Read the model definition and answer for the solid it produces. Units are mm, in the model's axes. Face numbers are marked on the shaded views. A direction names the side the tool comes from. Coordinates: 2 decimals unless noted, no trailing zeros. Write each loop counter-clockwise with the first axis right and the second up, starting at its lowest first coordinate (ties: lowest second). Pieces come first, ordered by that corner, then holes.
Item 1: Section A-A (y = 0) is taken. Give the vertices of the cut face in (x, z) (3 decimals).
Item 2: Section D-D (y = 10.5) is taken. Give the vertices of the cut face in (x, z).
Item 3: Section B-B (x = -9) is taken. Give the vertices of the cut face in (y, z), then the cut area to 3 significant figures.
Item 4: Each of these flat-tipped pins is pushed along its axis until it touches: P1, Ø8, axis at x = -6, y = -6, coming from the +Z side; P2, Ø4, axis at x = -0.5, z = 15, coming from the +Y side (3 decimals); P3, Ø1.5, axis at y = -4, z = -22.5, coming from the -X side; P4, Ø4, axis at x = -23.5, y = 23.5, coming from the -Z side. Where does it stop, or does it pass through?
Item 5: A tool of negligible diameter and unlimited length cuts with its end or side. For the marked faces 1 and 2, from which of +Z, -Z, +X, -X, +Y, -Y can it reach the whole face along a straight path? Write none if from no direction.
Item 6: Straight lines are drawn through the part: probe 1 along Y at (x, z) = (23.5, -2.85); probe 2 along Y at (x, z) = (-23, -2). For each, find the intervals that lie inside material, in ascending order.
Item 7: Section C-C (x = 0) is taken. Give the vertices of the cut face in (y, z) (3 decimals), then the cut area to 3 significant figures.
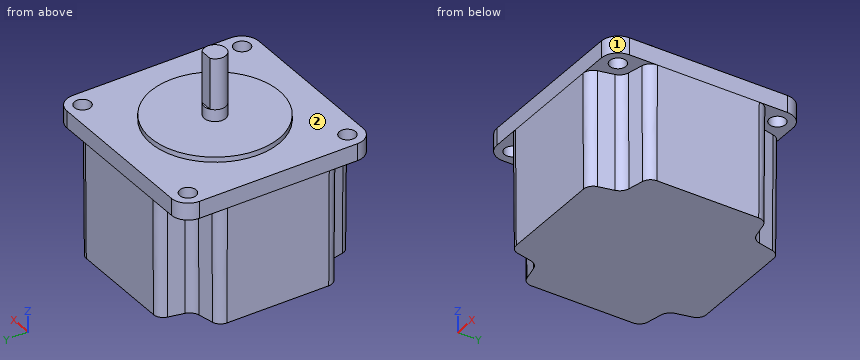
from build123d import *

# Parameters (mm, degrees)
F0_W      = 56.5
F0_H      = 56.5
F1_DEPTH  = 5
F3_DEPTH  = 34
F3_TAPER  = 0.4
F4_R      = 2.4
F5_DEPTH  = 5
F6_R      = 5
F7_R      = 19
F8_DEPTH  = 1.5
F9_R      = 3.175
F10_DEPTH = 3.5
F12_DEPTH = 15


with BuildPart() as f1:
    # F0 (on Top) → F1 (new body)
    with BuildSketch(Plane.XY):
        Rectangle(F0_W, F0_H)
    extrude(amount=-F1_DEPTH)

    # F2 (on face) → F3 (join)
    with BuildSketch(Plane(origin=(0, 0, -5), x_dir=(1, 0, 0), z_dir=(0, 0, -1))):
        with BuildLine():
            Line((15, 28.25), (0, 28.25))
            Line((0, 28.25), (-15, 28.25))
            ThreePointArc((-15, 28.25), (-16.9232649975, 27.5737223332), (-18, 25.842554673))
            Line((-18, 25.842554673), (-19, 21.3345213365))
            ThreePointArc((-19, 21.3345213365), (-19.8271146082, 19.8271146082), (-21.3345213365, 19))
            Line((-21.3345213365, 19), (-25.842554673, 18))
            ThreePointArc((-25.842554673, 18), (-27.5737223332, 16.9232649975), (-28.25, 15))
            Line((-28.25, 15), (-28.25, 0))
            Line((-28.25, 0), (-28.25, -15))
            ThreePointArc((-28.25, -15), (-27.5737223332, -16.9232649975), (-25.842554673, -18))
            Line((-25.842554673, -18), (-21.3345213365, -19))
            ThreePointArc((-21.3345213365, -19), (-19.8271146082, -19.8271146082), (-19, -21.3345213365))
            Line((-19, -21.3345213365), (-18, -25.842554673))
            ThreePointArc((-18, -25.842554673), (-16.9232649975, -27.5737223332), (-15, -28.25))
            Line((-15, -28.25), (0, -28.25))
            Line((0, -28.25), (15, -28.25))
            ThreePointArc((15, -28.25), (16.9232649975, -27.5737223332), (18, -25.842554673))
            Line((18, -25.842554673), (19, -21.3345213365))
            ThreePointArc((19, -21.3345213365), (19.8271146082, -19.8271146082), (21.3345213365, -19))
            Line((21.3345213365, -19), (25.842554673, -18))
            ThreePointArc((25.842554673, -18), (27.5737223332, -16.9232649975), (28.25, -15))
            Line((28.25, -15), (28.25, 0))
            Line((28.25, 0), (28.25, 15))
            ThreePointArc((28.25, 15), (27.5737223332, 16.9232649975), (25.842554673, 18))
            Line((25.842554673, 18), (21.3345213365, 19))
            ThreePointArc((21.3345213365, 19), (19.8271146082, 19.8271146082), (19, 21.3345213365))
            Line((19, 21.3345213365), (18, 25.842554673))
            ThreePointArc((18, 25.842554673), (16.9232649975, 27.5737223332), (15, 28.25))
        make_face()
    extrude(amount=F3_DEPTH, taper=F3_TAPER)

    # F4 (on face) → F5 (cut, through all)
    with BuildSketch(Plane.XY):
        with Locations((-23.5, 23.5)):
            Circle(F4_R)
        with Locations((23.5, 23.5)):
            Circle(F4_R)
        with Locations((-23.5, -23.5)):
            Circle(F4_R)
        with Locations((23.5, -23.5)):
            Circle(F4_R)
    extrude(amount=-F5_DEPTH, mode=Mode.SUBTRACT)

    # F6
    f6_edges = [f1.edges().sort_by_distance(p)[0] for p in [
        (28.25, 28.25, -2.5),
        (-28.25, 28.25, -2.5),
        (-28.25, -28.25, -2.5),
        (28.25, -28.25, -2.5),
    ]]
    fillet(f6_edges, radius=F6_R)

    # F7 (on face) → F8 (join)
    with BuildSketch(Plane.XY):
        Circle(F7_R)
    extrude(amount=F8_DEPTH)

    # F9 (on face) → F10 (join)
    with BuildSketch(Plane.XY.offset(1.5)):
        Circle(F9_R)
    extrude(amount=F10_DEPTH)

    # F11 (on face) → F12 (join)
    with BuildSketch(Plane.XY.offset(5)):
        with BuildLine():
            Line((1.7860571099, 2.625), (-1.7860571099, 2.625))
            ThreePointArc((-1.7860571099, 2.625), (0, -3.175), (1.7860571099, 2.625))
        make_face()
    extrude(amount=F12_DEPTH)


solid = f1.part
Established:
1. outline: (-28.25, -5) - (-28.013, -39) - (28.013, -39) - (28.25, -5) - (28.25, 0) - (19, 0) - (19, 1.5) - (3.175, 1.5) - (3.175, 20) - (-3.175, 20) - (-3.175, 1.5) - (-19, 1.5) - (-19, 0) - (-28.25, 0) - close
2. outline: (-28.25, -5) - (-28.01, -39) - (28.01, -39) - (28.25, -5) - (28.25, 0) - (15.84, 0) - (15.84, 1.5) - (-15.84, 1.5) - (-15.84, 0) - (-28.25, 0) - close
3. outline: (-28.25, -5) - (-28.01, -39) - (28.01, -39) - (28.25, -5) - (28.25, 0) - (16.73, 0) - (16.73, 1.5) - (-16.73, 1.5) - (-16.73, 0) - (-28.25, 0) - close
3. area: 2,250 mm2
4. P1: stops at z = 1.5
4. P2: stops at y = 2.625
4. P3: stops at x = -28.13
4. P4: passes through
5. face 1: +Z, -Z, +X, -Y
5. face 2: +Z
6. probe 1: y = -28.24 to -25.9, -21.1 to 21.1, 25.9 to 28.24
6. probe 2: y = -28.25 to -25.85, -21.15 to 21.15, 25.85 to 28.25
7. outline: (-28.25, -5) - (-28.013, -39) - (28.013, -39) - (28.25, -5) - (28.25, 0) - (19, 0) - (19, 1.5) - (3.175, 1.5) - (3.175, 5) - (2.625, 5) - (2.625, 20) - (-3.175, 20) - (-3.175, 1.5) - (-19, 1.5) - (-19, 0) - (-28.25, 0) - close
7. area: 2,360 mm2
